For this review, take the finished solid that the model builds, in its own axes (mm). Face numbers are marked on the shaded views. A direction names the side the tool comes from. Coordinates: 2 decimals unless noted, no trailing zeros. Write each loop counter-clockwise with the first axis right and the second up, starting at its lowest first coordinate (ties: lowest second). Pieces come first, ordered by that corner, then holes.
1) Insertion check: P1, Ø3, axis at x = -1.5, y = 7.5, coming from the -Z side; P2, Ø1.5, axis at y = 23.5, z = -1, coming from the -X side; P3, Ø1.2, axis at x = 0.5, y = 13.5, coming from the +Z side. Each pin has a flat end and moves straight along its axis. Give the tip position at first contact, or say it passes through.
2) We need section D-D on x = 1.5. Write out the cut boundary in (y, z).
3) To check wall thickness, follow line 1 along Y through (x, z) = (0.75, 2.25); line 2 along Y through (x, z) = (3, -1.75); line 3 along X through (y, z) = (-2, 0). State the ranges of each line that lie inside material, in increasing order.
4) We need section A-A on x = -1.25. Write out the cut boundary in (y, z).
5) We need section C-C on y = 10.5. Write out the cut boundary in (x, z), then the cut area to 3 significant figures.
6) We need section B-B on z = -1.75. Write out the cut boundary in (x, y).
7) For the marked faces 1 and 2, list the 3-axis set-ups (+Z, -Z, +X, -X, +Y, -Y) from which the entire face can be reached by the end or side of a thin tool; tool diameter is ignored.
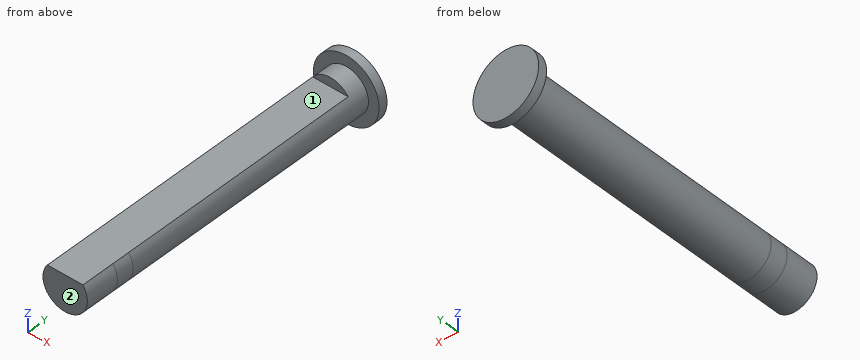
from build123d import *

# Parameters (mm, degrees)
EXTRUDE_1_DEPTH = 27.8
SKETCH_2_R      = 2.5
EXTRUDE_2_DEPTH = 2
SKETCH_3_R      = 3.7
EXTRUDE_3_DEPTH = 1
EXTRUDE_4_DEPTH = 2
EXTRUDE_5_DEPTH = 3.8


with BuildPart() as part:
    # 草图1 → 凸台-拉伸1 (new body)
    with BuildSketch(Plane(origin=(0, 0, 0), x_dir=(1, 0, 0), z_dir=(0, 1, 0))):
        with BuildLine():
            Line((-2, -1.5), (2, -1.5))
            ThreePointArc((2, -1.5), (0, 2.5), (-2, -1.5))
        make_face()
    extrude(amount=EXTRUDE_1_DEPTH)

    # 草图2 → 凸台-拉伸2 (add)
    with BuildSketch(Plane(origin=(0, 27.8, 0), x_dir=(1, 0, 0), z_dir=(0, 1, 0))):
        Circle(SKETCH_2_R)
    extrude(amount=EXTRUDE_2_DEPTH)

    # 草图3 → 凸台-拉伸3 (add)
    with BuildSketch(Plane(origin=(0, 29.8, 0), x_dir=(1, 0, 0), z_dir=(0, 1, 0))):
        Circle(SKETCH_3_R)
    extrude(amount=EXTRUDE_3_DEPTH)

    # 草图4 → 凸台-拉伸4 (add)
    with BuildSketch(Plane.XZ):
        with BuildLine():
            Line((-2, 1.5), (2, 1.5))
            ThreePointArc((2, 1.5), (0, -2.5), (-2, 1.5))
        make_face()
    extrude(amount=EXTRUDE_4_DEPTH)

    # 草图5 → 凸台-拉伸5 (add)
    with BuildSketch(Plane.XZ.offset(2)):
        with BuildLine():
            Line((-2, 1.5), (2, 1.5))
            ThreePointArc((2, 1.5), (0, -2.5), (-2, 1.5))
        make_face()
    extrude(amount=EXTRUDE_5_DEPTH)


solid = part.part
Result:
1. P1: stops at z = -2.5
1. P2: stops at x = -2.49
1. P3: stops at z = 1.5
2. outline: (-5.8, -2) - (29.8, -2) - (29.8, -3.38) - (30.8, -3.38) - (30.8, 3.38) - (29.8, 3.38) - (29.8, 2) - (27.8, 2) - (27.8, 1.5) - (-5.8, 1.5) - close
3. line 1: y = 27.8 to 30.8
3. line 2: y = 29.8 to 30.8
3. line 3: x = -2.5 to 2.5
4. outline: (-5.8, -2.17) - (29.8, -2.17) - (29.8, -3.48) - (30.8, -3.48) - (30.8, 3.48) - (29.8, 3.48) - (29.8, 2.17) - (27.8, 2.17) - (27.8, 1.5) - (-5.8, 1.5) - close
5. outline: (-2, 1.5) arc R2.5 ccw (long way) to (2, 1.5) - close
5. area: 16.8 mm2
6. outline: (-3.26, 29.8) - (-1.79, 29.8) - (-1.79, -5.8) - (1.79, -5.8) - (1.79, 29.8) - (3.26, 29.8) - (3.26, 30.8) - (-3.26, 30.8) - close
7. face 1: +Z, +X, -X, -Y
7. face 2: +Z, -Z, +X, -X, -Y
